Source: CAD feature listing. Evaluate the final solid. Frame: model axes, mm. Face numbers are marked on the shaded views. A direction names the side the tool comes from. Give positions to 0.01 mm unless a question says otherwise; leave off trailing zeros. Write each loop counter-clockwise with the first axis right and the second up, starting at its lowest first coordinate (ties: lowest second). Pieces come first, ordered by that corner, then holes. Notation, with made-up numbers: M 67,16.25 L 98,16.25 A20 ccw 98,25.25 Z; hole C 88.5,72 d11. An arc over 180 degrees is marked long. Return JSON: item names as keys, results as strings.
Autodesk Fusion 360 part; units mm, degrees
sketch "Sketch1" plane through (0, 0, 0) normal (0, 0, 1) x (1, 0, 0)
  circle A0 centre (0, 0) radius 50
extrude "Extrude1" add sketch "Sketch1" along normal blind 20
ref_plane "WorkPlane1" through (0, 0, 10) normal (0, 0, 1) x (1, 0, 0)
sketch "Sketch2" plane through (0, 0, 10) normal (0, 0, 1) x (1, 0, 0)
  circle A0 centre (0, 0) radius 47.5
extrude "Extrude2" cut sketch "Sketch2" along normal blind 10
sketch "Sketch3" plane through (0, 0, 0) normal (0, 0, 1) x (1, 0, 0)
  circle A0 centre (0, 0) radius 20
extrude "Extrude3" add sketch "Sketch3" against normal blind 20
sketch "Sketch4" plane through (0, 0, -20) normal (0, 0, -1) x (1, 0, 0)
  circle A0 centre (0, 0) radius 20
shell "Shell1" thickness 1 outward yes removed faces 1 at (6.3705, -1.965, -20)
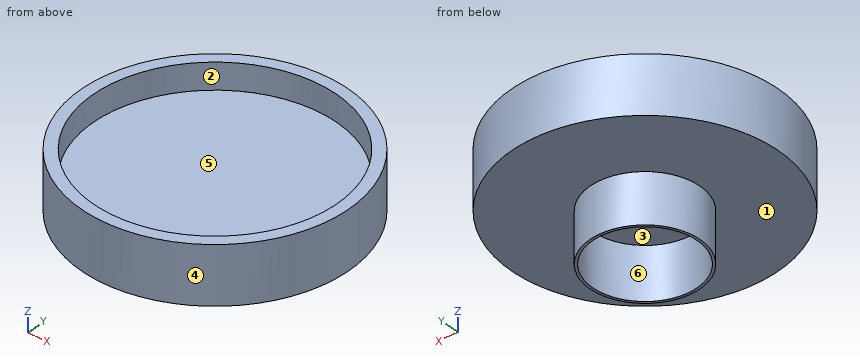
1) Line query: line 1 (Y direction, x = 0, z = 10.5); line 2 (Y direction, x = 0, z = 12); line 3 (Z direction, x = 11.5, y = 22.5). Output: solid intervals per line, ascending. Write a range as [from, to].
Numbers:
{"line 1": "y = [-51, -50], [-47.5, 47.5], [50, 51]", "line 2": "y = [-51, -50], [-47.5, -46.5], [46.5, 47.5], [50, 51]", "line 3": "z = [-1, 0], [10, 11]"}
2) Contact query for flat-ended pins moving along their axis: pin 1 Ø3 at (x, y) = (11.5, 14.5) entering from +Z; pin 2 Ø2 at (y, z) = (-14, -1.5) entering from -X; pin 3 Ø6 at (x, z) = (28.5, 13.5) entering from -Y. Output: stop coordinate, or through.
Numbers:
{"pin 1": "stops at z = 11", "pin 2": "stops at x = -49.28", "pin 3": "stops at y = -44.17"}
3) Cut plane D-D, the plane x = -23. Return the cut outline in (y, z).
Numbers:
{"outline": "M -45.52,-1 L 45.52,-1 L 45.52,21 L 40.41,21 L 40.41,11 L -40.41,11 L -40.41,21 L -45.52,21 Z; hole M -44.4,0 L 44.4,0 L 44.4,20 L 41.56,20 L 41.56,10 L -41.56,10 L -41.56,20 L -44.4,20 Z"}
4) Draft query along X for the marked faces 1, 2, 3 and 4. Return one class per face: released by +X, released by -X, zero draft, split by the parting line, or undercut.
Numbers:
{"face 1": "zero draft", "face 2": "undercut", "face 3": "undercut", "face 4": "split by the parting line"}
5) Set-up query: the marked faces 5 and 6. Return all of +Z, -Z, +X, -X, +Y, -Y with unobstructed straight access to the full face (end or side cutting, diameter ignored); none if empty.
Numbers:
{"face 5": "+Z", "face 6": "-Z"}
6) Cut plane A-A, the plane z = 17. Return the cut outline in (x, y), then the cut area to 3 significant figures.
Numbers:
{"outline": "C 0,0 d102; C 0,0 d95; hole C 0,0 d100; hole C 0,0 d93", "area": "613 mm²"}
7) Cut plane B-B, the plane x = 0. Return the cut outline in (y, z).
Numbers:
{"outline": "M -51,-1 L -21,-1 L -21,-20 L -20,-20 L -20,0 L -50,0 L -50,20 L -47.5,20 L -47.5,10 L 47.5,10 L 47.5,20 L 50,20 L 50,0 L 20,0 L 20,-20 L 21,-20 L 21,-1 L 51,-1 L 51,21 L 46.5,21 L 46.5,11 L -46.5,11 L -46.5,21 L -51,21 Z"}
